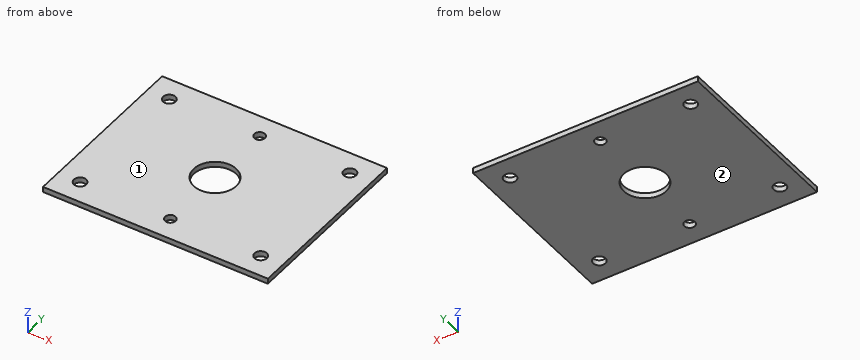
```python
from build123d import *

# Parameters (mm, degrees)
F0_W     = 254
F0_H     = 203
F0_R     = 7
F0_R_2   = 6
F0_R_3   = 24
F1_DEPTH = 6.1


with BuildPart() as f1:
    # F0 (on Top) → F1 (new body)
    with BuildSketch(Plane.XY):
        with Locations((127, 101.5)):
            Rectangle(F0_W, F0_H)
        with Locations((25, 25.5)):
            Circle(F0_R, mode=Mode.SUBTRACT)
        with Locations((127, 25.5)):
            Circle(F0_R_2, mode=Mode.SUBTRACT)
        with Locations((229, 25.5)):
            Circle(F0_R, mode=Mode.SUBTRACT)
        with Locations((25, 177.5)):
            Circle(F0_R, mode=Mode.SUBTRACT)
        with Locations((127, 101.5)):
            Circle(F0_R_3, mode=Mode.SUBTRACT)
        with Locations((127, 177.5)):
            Circle(F0_R_2, mode=Mode.SUBTRACT)
        with Locations((229, 177.5)):
            Circle(F0_R, mode=Mode.SUBTRACT)
    extrude(amount=F1_DEPTH)


solid = f1.part
```
Check sheet for the modelled part. Datum: model origin and axes. Units: mm. Face numbers are marked on the shaded views. Coordinates: 2 decimals unless noted, no trailing zeros. Order: outer loops, then holes, each group sorted by start corner. A loop starts at its lowest first (then second) coordinate and runs counter-clockwise, first axis right, second up. Notation, with made-up numbers: M 58,68.25 L 108,68.25 A6 cw 108,72.25 Z; hole C 13.25,37.25 d1. An arc over 180 degrees is marked long. Write each question's results on one line, items separated by ' | '. Start each with the question number.
1. Mould release check, pull along Z, two halves, no side actions. Record for the marked faces 1 and 2: +Z half, -Z half, draft (parallel to the pull), parting line (faces both ways), or undercut.
2. Cross-section at A-A on x = 229. Record the cut outline in (y, z).
3. Material ranges on probe 1 along Y at (x, z) = (127, 4.25); probe 2 along Y at (x, z) = (25, 2.5); probe 3 along Y at (x, z) = (119, 4.25), recorded low to high.
4. Cross-section at D-D on x = 127. Record the cut outline in (y, z).
5. Go/stop test with a flat-tipped pin: P1, Ø11, axis at x = 229, y = 25.5, coming from the +Z side. Record where the tip stops, or that it passes through.
6. Cross-section at C-C on z = 2.5. Record the cut outline in (x, y).
7. Cross-section at B-B on y = 25.5. Record the cut outline in (x, z).
Checks:
1) face 1: +Z half | face 2: -Z half
2) outline: M 0,0 L 18.5,0 L 18.5,6.1 L 0,6.1 Z; M 32.5,0 L 170.5,0 L 170.5,6.1 L 32.5,6.1 Z; M 184.5,0 L 203,0 L 203,6.1 L 184.5,6.1 Z
3) probe 1: y = 0 to 19.5, 31.5 to 77.5, 125.5 to 171.5, 183.5 to 203 | probe 2: y = 0 to 18.5, 32.5 to 170.5, 184.5 to 203 | probe 3: y = 0 to 78.87, 124.13 to 203
4) outline: M 0,0 L 19.5,0 L 19.5,6.1 L 0,6.1 Z; M 31.5,0 L 77.5,0 L 77.5,6.1 L 31.5,6.1 Z; M 125.5,0 L 171.5,0 L 171.5,6.1 L 125.5,6.1 Z; M 183.5,0 L 203,0 L 203,6.1 L 183.5,6.1 Z
5) P1: passes through
6) outline: M 0,0 L 254,0 L 254,203 L 0,203 Z; hole C 25,25.5 d14; hole C 25,177.5 d14; hole C 127,101.5 d48; hole C 127,25.5 d12; hole C 127,177.5 d12; hole C 229,25.5 d14; hole C 229,177.5 d14
7) outline: M 0,0 L 18,0 L 18,6.1 L 0,6.1 Z; M 32,0 L 121,0 L 121,6.1 L 32,6.1 Z; M 133,0 L 222,0 L 222,6.1 L 133,6.1 Z; M 236,0 L 254,0 L 254,6.1 L 236,6.1 Z
